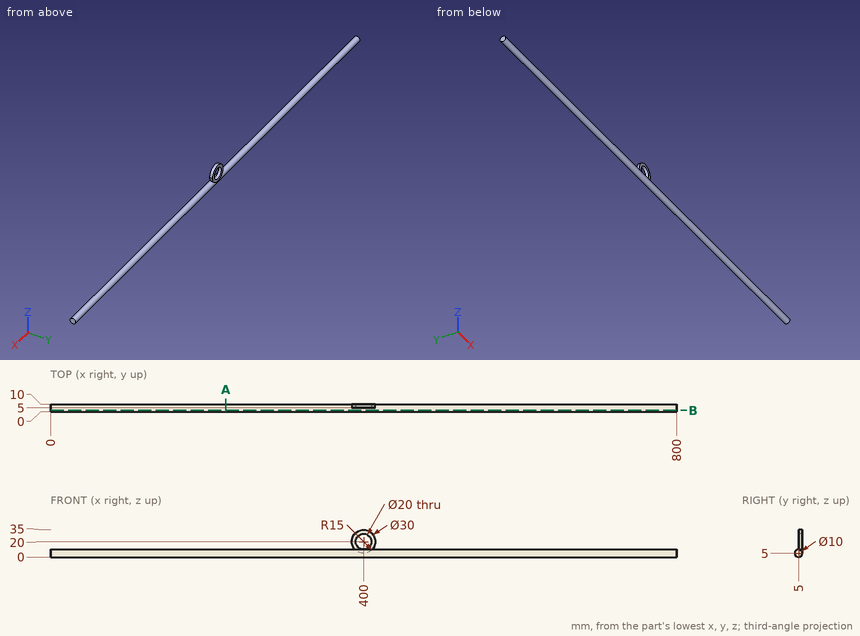
Job drawing, mm, ordinate dimensions from the low corner. One solid piece. Give positions to 0.01 mm unless a question says otherwise; leave off trailing zeros. Order: outer loops, then holes, each group sorted by start corner. A loop starts at its lowest first (then second) coordinate and runs counter-clockwise, first axis right, second up. Notation, with made-up numbers: (-0.5, 64) - (54.5, 64) arc R13 ccw to (54.5, 79) - close; hole circle Ø6 at (85.5, 49.5). An arc over 180 degrees is marked (long way). Answer in a Markdown table with one row per item.
1. Probe probe 1 along Z at (x, y) = (33.5, 4); probe 2 along Z at (x, y) = (540.5, 5.5); probe 3 along X at (y, z) = (9, 23.5). List the from-to ranges inside material, lowest first. Write a range as [from, to].
Data:
| item | result |
|---|---|
| probe 1 | z = [0.1, 9.9] |
| probe 2 | z = [0.03, 9.97] |
| probe 3 | x = [385.41, 390.63], [409.37, 414.59] |
2. Saw through at B-B, the plane y = 2. Give the cut face in (x, z).
Data:
| item | result |
|---|---|
| outline | (0, 1) - (800, 1) - (800, 9) - (0, 9) - close |
3. Saw through at A-A, the plane x = 224. Give the cut face in (y, z), plus the area to 3 significant figures.
Data:
| item | result |
|---|---|
| outline | circle Ø10 at (5, 5) |
| area | 78.5 mm² |
4. Flat gauge pins, fed straight in: pin 1 (5 mm diameter, centred on x = 253, z = 8, fed in from -Y); pin 2 (20 mm diameter, centred on x = 403, z = 23.5, fed in from -Y); pin 3 (2 mm diameter, centred on y = 6.5, z = 11.5, fed in from -X). Where does each tip first touch, or does it go through?
Data:
| item | result |
|---|---|
| pin 1 | stops at y = 0.03 |
| pin 2 | stops at y = 5 |
| pin 3 | stops at x = 387.01 |
